```python
from build123d import *

# Parameters (mm, degrees)
ESQUISSE1_W          = 83
ESQUISSE1_H          = 27
BOSS_EXTRU_1_DEPTH   = 1.75
D_PLACER_LA_FACE1_BY = 2
ESQUISSE3_W          = 2
ESQUISSE3_H          = 27
BOSS_EXTRU_3_DEPTH   = 3


with BuildPart() as part:
    # Esquisse1 → Boss.-Extru.1 (new body)
    with BuildSketch(Plane.XY):
        with Locations((-41.5, 13.5)):
            Rectangle(ESQUISSE1_W, ESQUISSE1_H)
    extrude(amount=BOSS_EXTRU_1_DEPTH)

    # Déplacer la face1: a face moved outward by 2.0
    extrude(part.faces().sort_by_distance((0, 13.5, 0.875))[0], amount=D_PLACER_LA_FACE1_BY, dir=(1, 0, 0))

    # Esquisse3 → Boss.-Extru.3 (add)
    with BuildSketch(Plane(origin=(0, 0, 0), x_dir=(-1, 0, 0), z_dir=(0, 0, -1))):
        with Locations((-1, 13.5)):
            Rectangle(ESQUISSE3_W, ESQUISSE3_H)
    extrude(amount=BOSS_EXTRU_3_DEPTH)


solid = part.part
```
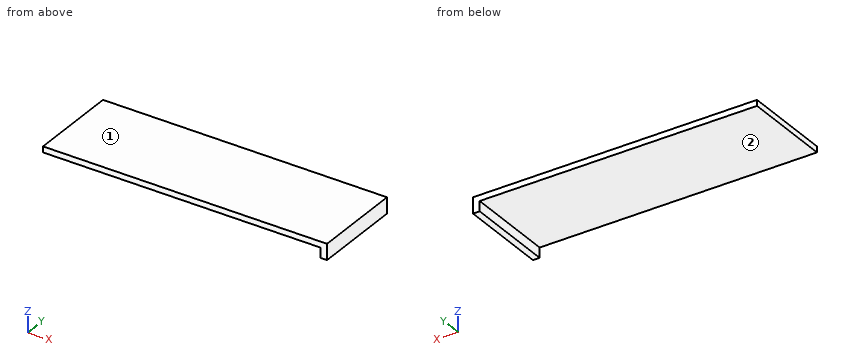
Could you check a few things on this model? Use its own coordinates, in mm. Face numbers are marked on the shaded views. A direction names the side the tool comes from. Coordinates: 2 decimals unless noted, no trailing zeros. Order: outer loops, then holes, each group sorted by start corner. A loop starts at its lowest first (then second) coordinate and runs counter-clockwise, first axis right, second up. Notation, with made-up numbers: M 13,-22.5 L 36,-22.5 A12 cw 36,-10.5 Z; hole C 80,37 d2. An arc over 180 degrees is marked long. Use a Markdown table: item, result. Add a question column.
Q1. I want a section at C-C on x = -22. List the corners of the cut face in (y, z) for me.
Q2. I want a section at B-B on z = -1.45. List the corners of the cut face in (x, y) for me.
Q3. Which directions (+Z, -Z, +X, -X, +Y, -Y) give clear straight access to the entire face, cutting with the end or side of a thin tool? Please do the marked faces 1 and 2.
Q4. I want a section at A-A on y = 14.75. List the corners of the cut face in (x, z) for me, then the cut area to 3 significant figures.
Q5. If I drill on L1, parallel to Z at x = -51, y = 16.5; L2, parallel to X at y = 8.5, z = -1.85, over which ranges is the centre line in solid material (lowest first)?
Q6. I'm going to push a flat-ended pin straight in: pin 1 (10 mm diameter, centred on x = -57, y = 20.5, fed in from -Z). Where does the tip first touch, or does it pass through?
Checked values:
| question | item | result |
|---|---|---|
| 1 | outline | M 0,0 L 27,0 L 27,1.75 L 0,1.75 Z |
| 2 | outline | M 0,0 L 2,0 L 2,27 L 0,27 Z |
| 3 | face 1 | +Z, +X, -X, +Y, -Y |
| 3 | face 2 | -Z, -X, +Y, -Y |
| 4 | outline | M -83,0 L 0,0 L 0,-3 L 2,-3 L 2,1.75 L -83,1.75 Z |
| 4 | area | 155 mm² |
| 5 | L1 | 0 to 1.75 |
| 5 | L2 | 0 to 2 |
| 6 | pin 1 | z = 0 |
